from build123d import *

# Parameters (mm, degrees)
SKETCH1_W           = 43.9
SKETCH1_H           = 20.5
BOSS_EXTRUDE1_DEPTH = 16.5
SKETCH3_R           = 1.6
CUT_EXTRUDE1_DEPTH  = 6.5
SKETCH5_W           = 35.96646031
SKETCH5_H           = 15.929900813
CUT_EXTRUDE3_DEPTH  = 12.5
SKETCH4_W           = 12.608694843
SKETCH4_H           = 15.64948953
SKETCH4_W_2         = 13.340907584
CUT_EXTRUDE4_DEPTH  = 28.5
SKETCH6_R           = 0.45
BOSS_EXTRUDE2_DEPTH = 3.5


with BuildPart() as part:
    # Sketch1 → Boss-Extrude1 (new body)
    with BuildSketch(Plane(origin=(0, 0, 0), x_dir=(1, 0, 0), z_dir=(0, 1, 0))):
        with Locations((-0.724764151, -1.035141509)):
            Rectangle(SKETCH1_W, SKETCH1_H)
    extrude(amount=BOSS_EXTRUDE1_DEPTH)

    # Sketch3 → Cut-Extrude1 (cut)
    with BuildSketch(Plane(origin=(0, 0, 0), x_dir=(-1, 0, 0), z_dir=(0, -1, 0))):
        with Locations((-13.145235849, -1.035141509)):
            Circle(SKETCH3_R)
        with Locations((14.594764151, -1.035141509)):
            Circle(SKETCH3_R)
    extrude(amount=-CUT_EXTRUDE1_DEPTH, mode=Mode.SUBTRACT)

    # Sketch5 → Cut-Extrude3 (cut)
    with BuildSketch(Plane(origin=(0, 16.5, 0), x_dir=(1, 0, 0), z_dir=(0, 1, 0))):
        with Locations((-0.591045911, -0.805962597)):
            Rectangle(SKETCH5_W, SKETCH5_H)
    extrude(amount=-CUT_EXTRUDE3_DEPTH, mode=Mode.SUBTRACT)

    # Sketch4 → Cut-Extrude4 (cut)
    with BuildSketch(Plane(origin=(0, 0, -9.214858491), x_dir=(-1, 0, 0), z_dir=(0, 0, -1))):
        with Locations((-8.682774774, 12.932468191)):
            Rectangle(SKETCH4_W, SKETCH4_H)
        with Locations((11.03272818, 12.932468191)):
            Rectangle(SKETCH4_W_2, SKETCH4_H)
    extrude(amount=-CUT_EXTRUDE4_DEPTH, mode=Mode.SUBTRACT)

    # Sketch6 → Boss-Extrude2 (add)
    with BuildSketch(Plane.XZ):
        with Locations((20.765235849, 1.035141509)):
            Circle(SKETCH6_R)
        with Locations((-22.214764151, 1.035141509)):
            Circle(SKETCH6_R)
    extrude(amount=BOSS_EXTRUDE2_DEPTH)


solid = part.part
CAD build for the part. Positions are in the model's coordinates, mm. A direction names the side the tool comes from. Coordinates: 2 decimals unless noted, no trailing zeros. Write each loop counter-clockwise with the first axis right and the second up, starting at its lowest first coordinate (ties: lowest second). Pieces come first, ordered by that corner, then holes. Notation, with made-up numbers: (-38.5, 70.5) - (0.5, 70.5) arc R32 ccw to (0.5, 109.5) - close; hole circle Ø9 at (-32.75, 20.5). An arc over 180 degrees is marked (long way). Use a Markdown table: item, result. Add a question column.
Item 1: Mould opens along X. For faces 6 (the face through (21.225, 8, 1)), 7 (the face through (-22.664, -1.726, 1.055)), 8 (the face through (-1, 16.5, 10)) say: pulls with the +X half, pulls with the -X half, needs draft (parallel to the pull), parting line crosses it, or undercut.
Item 2: 3-axis set-ups, long thin cutter, end or side, ignore diameter. For faces 1 (the face through (-12.996, 1.972, 0.965)), 2 (the face through (-22.675, 8, 1)), 3 (the face through (1, 9, -7.159)), 4 (the face through (20.316, -1.726, 1.055)), 5 (the face through (-17.703, 11, -8)): which of +Z, -Z, +X, -X, +Y, -Y reach the whole face in a straight line?
Item 3: Band-saw the part on C-C, the plane x = -5. Give the cut face in (y, z).
Item 4: Band-saw the part on A-A, the plane y = 11. Give the cut face in (x, z), and give its area (3 significant figures).
Item 5: Band-saw the part on B-B, the plane z = 8. Give the cut face in (x, y), and give its area (3 significant figures).
Item 6: Drill centre lines: L1, parallel to X at y = 7.5, z = 4.5; L2, parallel to Z at x = -15, y = 4.75; L3, parallel to Y at x = 13, z = 9.5. Where is each one in solid material? Low to high. Write a range as from..to.
Item 7: Band-saw the part on D-D, the plane y = 2. Give the cut face in (x, z), and give its area (3 significant figures).
Item 8: Flat gauge pins, fed straight in: pin 1 (1 mm diameter, centred on x = 3.5, y = 11.5, fed in from +Z); pin 2 (0.8 mm diameter, centred on x = -13.5, z = 10.5, fed in from +Y); pin 3 (3.5 mm diameter, centred on x = -14.59, z = 1.04, fed in from +Y). Where does each tip first touch, or does it go through?
Numbers:
| question | item | result |
|---|---|---|
| 1 | face 6 | pulls with the +X half |
| 1 | face 7 | undercut |
| 1 | face 8 | needs draft |
| 2 | face 1 | +Y, -Y |
| 2 | face 2 | +Z, -Z, -X, +Y, -Y |
| 2 | face 3 | +Y |
| 2 | face 4 | -Y |
| 2 | face 5 | +Z, -Z, +Y |
| 3 | outline | (0, -9.21) - (5.11, -9.21) - (5.11, -7.16) - (4, -7.16) - (4, 8.77) - (5.11, 8.77) - (5.11, 11.29) - (0, 11.29) - close |
| 4 | outline | (-22.67, -9.21) - (-17.7, -9.21) - (-17.7, -7.16) - (-18.57, -7.16) - (-18.57, 8.77) - (-17.7, 8.77) - (-17.7, 11.29) - (-22.67, 11.29) - close; (-4.36, -9.21) - (2.38, -9.21) - (2.38, -7.16) - (-4.36, -7.16) - close; (-4.36, 8.77) - (2.38, 8.77) - (2.38, 11.29) - (-4.36, 11.29) - close; (14.99, -9.21) - (21.23, -9.21) - (21.23, 11.29) - (14.99, 11.29) - (14.99, 8.77) - (17.39, 8.77) - (17.39, -7.16) - (14.99, -7.16) - close |
| 4 | area | 208 mm2 |
| 5 | outline | (-22.67, 0) - (21.23, 0) - (21.23, 16.5) - (17.39, 16.5) - (17.39, 4) - (-18.57, 4) - (-18.57, 16.5) - (-22.67, 16.5) - close |
| 5 | area | 275 mm2 |
| 6 | L1 | -22.67..-18.57, 17.39..21.23 |
| 6 | L2 | -9.21..-7.16, 8.77..11.29 |
| 6 | L3 | 0..5.11 |
| 7 | outline | (-22.67, -9.21) - (21.23, -9.21) - (21.23, 11.29) - (-22.67, 11.29) - close; hole circle Ø3.2 at (-14.59, 1.04); hole circle Ø3.2 at (13.15, 1.04) |
| 7 | area | 884 mm2 |
| 8 | pin 1 | through |
| 8 | pin 2 | y = 5.11 |
| 8 | pin 3 | y = 4 |
